from build123d import *

# Parameters (mm, degrees)
F0_R     = 15.875
F1_DEPTH = 50.8
F2_DEPTH = 76.2


with BuildPart() as f1:
    # F0 (on Top) → F1 (new body)
    with BuildSketch(Plane.XY):
        with BuildLine():
            Line((-11.237637, 36.40228), (-84.859044, 36.40228))
            ThreePointArc((-84.859044, 36.40228), (-62.408403, 27.10292), (-53.109044, 4.65228))
            ThreePointArc((-53.109044, 4.65228), (-62.408403, -17.79836), (-84.859044, -27.09772))
            Line((-84.859044, -27.09772), (-11.237637, -27.09772))
            Line((-11.237637, -27.09772), (62.38377, -27.09772))
            ThreePointArc((62.38377, -27.09772), (94.13377, 4.65228), (62.38377, 36.40228))
            Line((62.38377, 36.40228), (-11.237637, 36.40228))
        make_face()
        with Locations((62.38377, 4.65228)):
            Circle(F0_R, mode=Mode.SUBTRACT)
    extrude(amount=F1_DEPTH)

    # F0 (on Top) → F2 (join)
    with BuildSketch(Plane.XY):
        with BuildLine():
            ThreePointArc((-53.109044, 4.65228), (-62.408403, 27.10292), (-84.859044, 36.40228))
            ThreePointArc((-84.859044, 36.40228), (-116.609044, 4.65228), (-84.859044, -27.09772))
            ThreePointArc((-84.859044, -27.09772), (-62.408403, -17.79836), (-53.109044, 4.65228))
        make_face()
        with Locations((-84.859044, 4.65228)):
            Circle(F0_R, mode=Mode.SUBTRACT)
    extrude(amount=F2_DEPTH)


solid = f1.part
Can you work these out from the model? Positions are in its coordinate system, mm. Give positions to 0.01 mm unless a question says otherwise; leave off trailing zeros. Order: outer loops, then holes, each group sorted by start corner. A loop starts at its lowest first (then second) coordinate and runs counter-clockwise, first axis right, second up. Notation, with made-up numbers: (-4.5, 89.25) - (30.5, 89.25) arc R21 ccw to (30.5, 119.25) - close; hole circle Ø4 at (62.5, 44.5). An arc over 180 degrees is marked (long way). Write each question's results on one line, items separated by ' | '.
1) Suppose I cut it at C-C, the plane x = -79.5. Write out the boundary of the cut face in (y, z).
Final values:
outline: (-27.1, 0) - (-10.29, 0) - (-10.29, 76.2) - (-26.64, 76.2) - (-26.64, 50.8) - (-27.1, 50.8) - close; (19.6, 0) - (36.4, 0) - (36.4, 50.8) - (35.95, 50.8) - (35.95, 76.2) - (19.6, 76.2) - close
2) Suppose I cut it at B-B, the plane z = 7. Write out the boundary of the cut face in (x, y) (3 decimals), then the cut area to 3 significant figures.
Final values:
outline: (-84.859, -27.098) - (62.384, -27.098) arc R31.75 ccw to (62.384, 36.402) - (-84.859, 36.402) arc R31.75 ccw to start; hole circle Ø31.75 at (-84.859, 4.652); hole circle Ø31.75 at (62.384, 4.652) | area: 10,900 mm^2
3) Suppose I cut it at A-A, the plane y = 18.5. Write out the boundary of the cut face in (x, z).
Final values:
outline: (-113.43, 0) - (-92.62, 0) - (-92.62, 76.2) - (-113.43, 76.2) - close; (-77.1, 0) - (54.62, 0) - (54.62, 50.8) - (-56.29, 50.8) - (-56.29, 76.2) - (-77.1, 76.2) - close; (70.15, 0) - (90.95, 0) - (90.95, 50.8) - (70.15, 50.8) - close
4) If we mould it in two halves opening along X, with no side actions, what happens to faces 1 (the face through (-69.717, 9.421, 37.567)), 2 (the face through (94.126, 3.954, 25.044)), 3 (the face through (-10, 36.402, 25))? For each: pulls with the +X half, pulls with the -X half, needs draft (parallel to the pull), parting line crosses it, or undercut.
Final values:
face 1: undercut | face 2: pulls with the +X half | face 3: needs draft
5) Suppose I cut it at D-D, the plane z = 53.5. Write out the boundary of the cut face in (x, y) (3 decimals).
Final values:
outline: (-84.859, -27.098) arc R31.75 ccw to (-53.109, 4.652) arc R31.75 ccw (long way) to start; hole circle Ø31.75 at (-84.859, 4.652)
6) I'm going to push flat-ended pins straight in: pin 1 Ø2 at (y, z) = (11, 40) entering from +X; pin 2 Ø8 at (y, z) = (9.5, 36) entering from +X; pin 3 Ø2 at (y, z) = (-13, 24.5) entering from -X. Where does each tip first touch, or does it pass through?
Final values:
pin 1: stops at x = 93.68 | pin 2: stops at x = 94.12 | pin 3: stops at x = -111.89
7) Please list where these lines run through material, in increasing order: line 1 along X through (y, z) = (14, 17); line 2 along X through (y, z) = (0.5, 38); line 3 along Z through (x, y) = (37, 20.5). Write a range as [from, to].
Final values:
line 1: x = [-115.2, -97.69], [-72.03, 49.55], [75.21, 92.73] | line 2: x = [-116.34, -100.18], [-69.54, 47.06], [77.71, 93.86] | line 3: z = [0, 50.8]
